Could you check a few things on this drawing? It's one solid part, dimensions in mm from its lowest x, y, z. A direction names the side the tool comes from. Give positions to 0.01 mm unless a question says otherwise; leave off trailing zeros. Loops run counter-clockwise (first coordinate to the right, second up) from the corner with the lowest first, then second, coordinate; pieces in that order, holes last. Notation, with made-up numbers: (43, -27.5) - (52, -27.5) arc R13 cw to (52, -21.5) - close; hole circle Ø4 at (29, 55). An arc over 180 degrees is marked (long way). Write item = value, one per line.
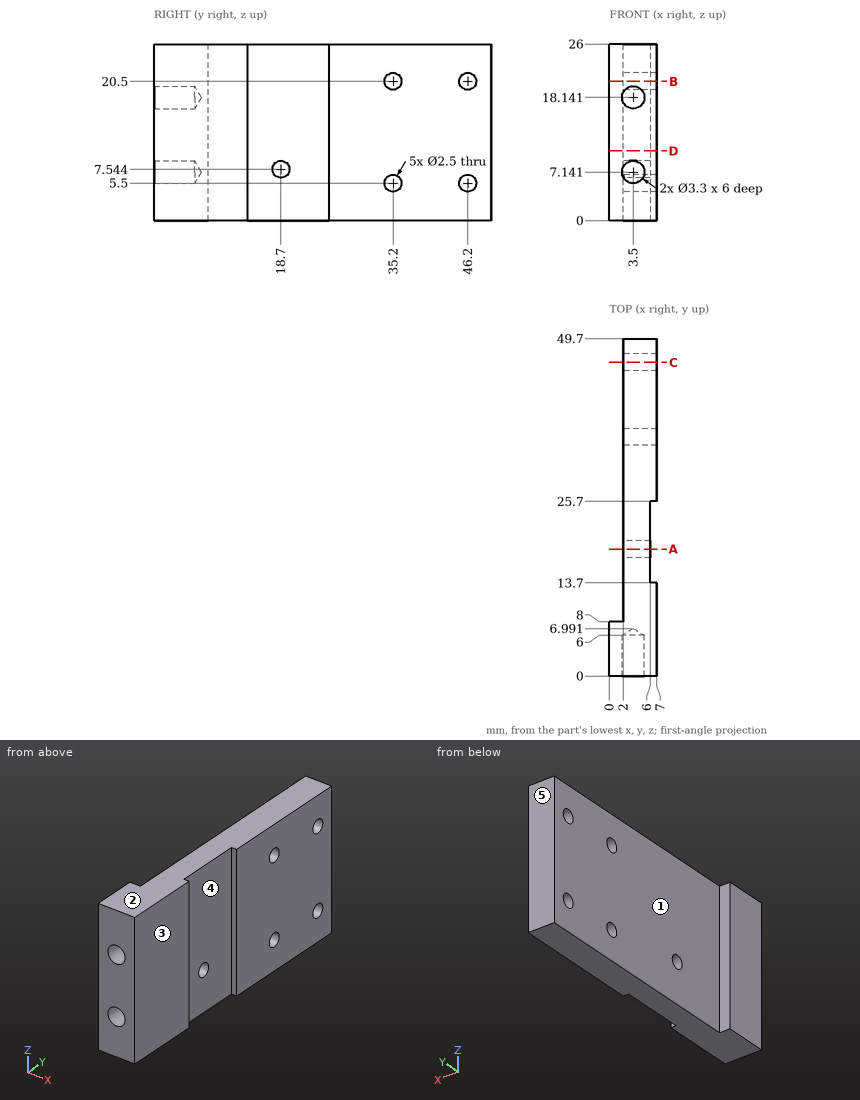
Q1. Imagine slicing it at D-D, the plane z = 10.25. Write out the boundary of the cut face in (x, y).
Output:
outline = (0, 0) - (7, 0) - (7, 13.7) - (6, 13.7) - (6, 25.7) - (7, 25.7) - (7, 49.7) - (2, 49.7) - (2, 8) - (0, 8) - close
Q2. Imagine slicing it at A-A, the plane y = 18.7. Write out the boundary of the cut face in (x, z) (1 decimal).
Output:
outline = (2, 0) - (6, 0) - (6, 6.3) - (2, 6.3) - close; (2, 8.8) - (6, 8.8) - (6, 26) - (2, 26) - close
Q3. Imagine slicing it at C-C, the plane y = 46.2. Write out the boundary of the cut face in (x, z), then the cut area to 3 significant figures.
Output:
outline = (2, 0) - (7, 0) - (7, 4.25) - (2, 4.25) - close; (2, 6.75) - (7, 6.75) - (7, 19.25) - (2, 19.25) - close; (2, 21.75) - (7, 21.75) - (7, 26) - (2, 26) - close
area = 105 mm2
Q4. We'd pull the mould along Y, two halves only. Please class the marked faces 3, 4 and 5: released by +Y, released by -Y, zero draft, split by the parting line, or undercut.
Output:
face_3 = zero draft
face_4 = undercut
face_5 = released by +Y
Q5. Imagine slicing it at B-B, the plane z = 20.5. Write out the boundary of the cut face in (x, y).
Output:
outline = (0, 0) - (7, 0) - (7, 13.7) - (6, 13.7) - (6, 25.7) - (7, 25.7) - (7, 33.95) - (2, 33.95) - (2, 8) - (0, 8) - close; (2, 36.45) - (7, 36.45) - (7, 44.95) - (2, 44.95) - close; (2, 47.45) - (7, 47.45) - (7, 49.7) - (2, 49.7) - close
Q6. I need wall thicknesses on L1, parallel to Y at x = 4.9, z = 20.5; L2, parallel to X at y = 21.5, z = 23.75; L3, parallel to X at y = 12.5, z = 24.5. Which ranges of each line are inside material? Lowest first, please.
Output:
L1 = 0 to 33.95, 36.45 to 44.95, 47.45 to 49.7
L2 = 2 to 6
L3 = 2 to 7
Q7. For pin 1 (1 mm diameter, centred on y = 26, z = 3.5, fed in from -X); pin 2 (2.5 mm diameter, centred on x = 3.5, z = 18.14, fed in from -Y), each with a flat end and sliding along its axis, tell me the tip position at first contact or that it passes through.
Output:
pin_1 = 2
pin_2 = 6.24
Q8. Which directions (+Z, -Z, +X, -X, +Y, -Y) give clear straight access to the entire face, cutting with the end or side of a thin tool? Please do the marked faces 1 and 2.
Output:
face_1 = +Z, -Z, -X, +Y
face_2 = +Z, +X, -X, +Y, -Y
